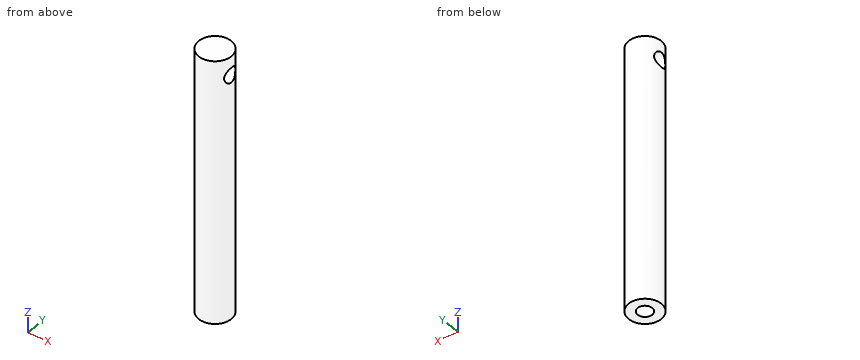
```python
from build123d import *

# Parameters (mm, degrees)
SKETCH1_W             = 5.5
SKETCH1_H             = 89
SKETCH2_R             = 2.5
CUT_EXTRUDE1_DEPTH    = 15
M6_TAPPED_HOLE1_D     = 4.891
M6_TAPPED_HOLE1_DEPTH = 30
M6_TAPPED_HOLE1_TIP   = 1.469404644


with BuildPart() as part:
    # Sketch1 → Revolve1 (revolve)
    with BuildSketch(Plane(origin=(0, 0, 0), x_dir=(1, 0, 0), z_dir=(0, 1, 0))):
        with Locations((2.75, 44.5)):
            Rectangle(SKETCH1_W, SKETCH1_H)
    revolve(axis=Axis((0, 0, 0), (0, 0, -1)))

    # Sketch2 → Cut-Extrude1 (cut, symmetric)
    with BuildSketch(Plane(origin=(0, 0, 0), x_dir=(0, 0, -1), z_dir=(1, 0, 0))):
        with Locations((6.35, 0)):
            Circle(SKETCH2_R)
    extrude(amount=CUT_EXTRUDE1_DEPTH, both=True, mode=Mode.SUBTRACT)

    # M6 Tapped Hole1
    with Locations(Plane(origin=(0, 0, -89), x_dir=(-1, 0, 0), z_dir=(0, 0, -1))):
        with Locations((0, 0)):
            Hole(M6_TAPPED_HOLE1_D / 2, depth=M6_TAPPED_HOLE1_DEPTH)
            with Locations((0, 0, -(M6_TAPPED_HOLE1_DEPTH + M6_TAPPED_HOLE1_TIP / 2))):  # 118° drill point
                Cone(0, M6_TAPPED_HOLE1_D / 2, M6_TAPPED_HOLE1_TIP, mode=Mode.SUBTRACT)


solid = part.part
```
Work out the finished part from the listing and answer in its coordinate system (mm). Give positions to 0.01 mm unless a question says otherwise; leave off trailing zeros. Order: outer loops, then holes, each group sorted by start corner. A loop starts at its lowest first (then second) coordinate and runs counter-clockwise, first axis right, second up. Notation, with made-up numbers: (59, -12) - (115, -12) arc R5 ccw to (115, -7) - close; hole circle Ø2 at (-35.75, 56.25). An arc over 180 degrees is marked (long way). One line per item, written item: value. Start each with the question number.
1. Section D-D, the plane z = -6.35 is taken. Write down the section's boundary in (x, y).
2. Consider line 1 (Y direction, x = 0, z = -6.35); line 2 (Z direction, x = 2.75, y = 0); line 3 (X direction, y = 0, z = -72). Determine where each line is inside the solid, lowest interval first.
3. Section A-A, the plane z = -71 is taken. Write down the section's boundary in (x, y).
4. Section C-C, the plane z = -34 is taken. Write down the section's boundary in (x, y).
5. Section B-B, the plane x = 4.75 is taken. Write down the section's boundary in (y, z), then the cut area to 3 significant figures.
6. Each of these flat-tipped pins is pushed along its axis until it touches: pin 1 Ø1.5 at (x, z) = (-3.5, -51.5) entering from +Y; pin 2 Ø4 at (y, z) = (-4, -29) entering from +X; pin 3 Ø1 at (x, z) = (2.5, -50) entering from +Y. Where does it stop, or does it pass through?
Filled sheet:
1. outline: (-4.9, -2.5) arc R5.5 ccw to (4.9, -2.5) - close; (-4.9, 2.5) - (4.9, 2.5) arc R5.5 ccw to start
2. line 1: -5.5 to -2.5, 2.5 to 5.5
2. line 2: -89 to -8.85, -3.85 to 0
2. line 3: -5.5 to -2.45, 2.45 to 5.5
3. outline: circle Ø11 at (0, 0); hole circle Ø4.89 at (0, 0)
4. outline: circle Ø11 at (0, 0)
5. outline: (-2.77, -89) - (2.77, -89) - (2.77, 0) - (-2.77, 0) - close; hole circle Ø5 at (0, -6.35)
5. area: 474 mm²
6. pin 1: y = 4.76
6. pin 2: x = 5.12
6. pin 3: y = 5.12
